from build123d import *

# Parameters (mm, degrees)
F0_W      = 3.175
F0_H      = 38.1
F1_DEPTH  = 23.8125
F0_W_2    = 38.1
F0_R      = 11.1125
F0_R_2    = 7.9375
F2_DEPTH  = 6.35
F4_D      = 4.4958
F5_D      = 4.4958
F6_D      = 4.4958
F7_D      = 4.4958
F8_D      = 4.4958
F9_D      = 4.4958
F10_DEPTH = 3.175


with BuildPart() as f1:
    # F0 (on Top) → F1 (new body)
    with BuildSketch(Plane.XY):
        with Locations((19.05, 0)):
            Rectangle(F0_W, F0_H)
    extrude(amount=F1_DEPTH)

    # F0 (on Top) → F2 (join)
    with BuildSketch(Plane.XY):
        with Locations((-1.5875, 0)):
            Rectangle(F0_W_2, F0_H)
        with Locations((-1.5875, 0)):
            Circle(F0_R, mode=Mode.SUBTRACT)
        with Locations((-1.5875, 0)):
            Circle(F0_R)
        with Locations((-1.5875, 0)):
            Circle(F0_R_2, mode=Mode.SUBTRACT)
    extrude(amount=F2_DEPTH)

    # F4 (through all)
    with Locations(Plane(origin=(0, 0, 0), x_dir=(1, 0, 0), z_dir=(0, 0, -1))):
        with Locations((-15.0622, 13.4747)):
            Hole(F4_D / 2)

    # F5 (through all)
    with Locations(Plane(origin=(0, 0, 0), x_dir=(1, 0, 0), z_dir=(0, 0, -1))):
        with Locations((-15.0622, -13.4747)):
            Hole(F5_D / 2)

    # F6 (through all)
    with Locations(Plane(origin=(0, 0, 0), x_dir=(1, 0, 0), z_dir=(0, 0, -1))):
        with Locations((11.8872, -13.4747)):
            Hole(F6_D / 2)

    # F7 (through all)
    with Locations(Plane(origin=(0, 0, 0), x_dir=(1, 0, 0), z_dir=(0, 0, -1))):
        with Locations((11.8872, 13.4747)):
            Hole(F7_D / 2)

    # F8 (through all)
    with Locations(Plane(origin=(17.4625, 0, 0), x_dir=(0, -1, 0), z_dir=(-1, 0, 0))):
        with Locations((-13.4747, 15.08125)):
            Hole(F8_D / 2)

    # F9 (through all)
    with Locations(Plane(origin=(17.4625, 0, 0), x_dir=(0, -1, 0), z_dir=(-1, 0, 0))):
        with Locations((13.4747, 15.08125)):
            Hole(F9_D / 2)

    # F0 (on Top) → F10 (cut)
    with BuildSketch(Plane.XY):
        with Locations((-1.5875, 0)):
            Circle(F0_R)
        with Locations((-1.5875, 0)):
            Circle(F0_R_2, mode=Mode.SUBTRACT)
    extrude(amount=F10_DEPTH, mode=Mode.SUBTRACT)


solid = f1.part
Could you check a few things on this model? Use its own coordinates, in mm. A direction names the side the tool comes from. Round coordinates to 2 decimals unless told otherwise and drop trailing zeros. Write each loop counter-clockwise with the first axis right and the second up, starting at its lowest first coordinate (ties: lowest second). Pieces come first, ordered by that corner, then holes. Notation, with made-up numbers: (-30.75, -11) -> (25.25, -11) arc R23 cw to (25.25, 23) -> close; hole circle Ø4 at (70, 49.25). An arc over 180 degrees is marked (long way). Use a Markdown table: item, result.
1. For pin 1 Ø1.5 at (x, y) = (-9.5, -6) entering from -Z (3 decimals); pin 2 Ø11.5 at (x, y) = (0.5, -7.5) entering from +Z; pin 3 Ø3.5 at (x, y) = (11.89, 13.47) entering from +Z; pin 4 Ø5 at (y, z) = (8.5, 10.5) entering from -X, each with a flat end and sliding along its axis, tell me the tip position at first contact or that it passes through.
Answer key:
| item | result |
|---|---|
| pin 1 | stops at z = 3.175 |
| pin 2 | stops at z = 6.35 |
| pin 3 | passes through |
| pin 4 | stops at x = 17.46 |
2. If we section it at B-B (x = 0.5): List the corners of the cut face in (y, z) for me (3 decimals), then the cut area to 3 significant figures.
Answer key:
| item | result |
|---|---|
| outline | (-19.05, 0) -> (-10.915, 0) -> (-10.915, 3.175) -> (-7.658, 3.175) -> (-7.658, 6.35) -> (-19.05, 6.35) -> close; (7.658, 3.175) -> (10.915, 3.175) -> (10.915, 0) -> (19.05, 0) -> (19.05, 6.35) -> (7.658, 6.35) -> close |
| area | 124 mm^2 |
3. If we section it at D-D (x = 11): List the corners of the cut face in (y, z) for me, then the cut area to 3 significant figures.
Answer key:
| item | result |
|---|---|
| outline | (-19.05, 0) -> (-15.54, 0) -> (-15.54, 6.35) -> (-19.05, 6.35) -> close; (-11.41, 0) -> (11.41, 0) -> (11.41, 6.35) -> (-11.41, 6.35) -> close; (15.54, 0) -> (19.05, 0) -> (19.05, 6.35) -> (15.54, 6.35) -> close |
| area | 189 mm^2 |
4. If we section it at C-C (z = 14): List the corners of the cut face in (x, y) for me.
Answer key:
| item | result |
|---|---|
| outline | (17.46, -19.05) -> (20.64, -19.05) -> (20.64, -15.45) -> (17.46, -15.45) -> close; (17.46, -11.5) -> (20.64, -11.5) -> (20.64, 11.5) -> (17.46, 11.5) -> close; (17.46, 15.45) -> (20.64, 15.45) -> (20.64, 19.05) -> (17.46, 19.05) -> close |
5. Please list where these lines run through material, in increasing order: probe 1 along X at (y, z) = (-13, 6.25) (1 decimal); probe 2 along Y at (x, z) = (10, 2.5); probe 3 along Z at (x, y) = (-4.5, 16.5).
Answer key:
| item | result |
|---|---|
| probe 1 | x = -20.6 to -17.3, -12.9 to 9.7, 14.1 to 20.6 |
| probe 2 | y = -19.05 to -14.7, -12.25 to 12.25, 14.7 to 19.05 |
| probe 3 | z = 0 to 6.35 |
6. We'd pull the mould along Z, two halves only. Please class faces 1 (the face through (19.07, -11.33, 15.76)), 2 (the face through (19.07, 14.68, 16.98)), 3 (the face through (9, 5, 0)), 4 (the face through (9.811, -12.614, 3.219)): +Z half, -Z half, draft (parallel to the pull), parting line (faces both ways), or undercut.
Answer key:
| item | result |
|---|---|
| face 1 | undercut |
| face 2 | undercut |
| face 3 | -Z half |
| face 4 | draft |
7. Which directions (+Z, -Z, +X, -X, +Y, -Y) give clear straight access to the entire face, cutting with the end or side of a thin tool? Please do faces 5 (the face through (-9.78, 7.51, 1.57)), 6 (the face through (-20.638, 0, 3)), 7 (the face through (17.463, 0, 15)).
Answer key:
| item | result |
|---|---|
| face 5 | -Z |
| face 6 | +Z, -Z, -X, +Y, -Y |
| face 7 | +Z, -X, +Y, -Y |
